```python
from build123d import *
from build123d.topology import SkipClean

# Parameters (mm, degrees)
EXTRUDE_1_DEPTH          = 3
EXTRUDE_3_DEPTH          = 5
EXTRUDE_3_DEPTH_BACK     = 5
SKETCH_5_R               = 6.36543
SKETCH_5_R_2             = 5.5
CUT_EXTRUDE_1_DEPTH      = 14
CUT_EXTRUDE_2_DEPTH      = 15.974979
CUT_EXTRUDE_2_DEPTH_BACK = 15.974979
SKETCH_6_R               = 0.975
SKETCH_7_R               = 3
SKETCH_7_R_2             = 0.9
EXTRUDE_4_DEPTH          = 7.5
CUT_EXTRUDE_3_DEPTH      = 1.45
CUT_EXTRUDE_3_DEPTH_BACK = 1.45
SKETCH_10_R              = 1.825
SKETCH_10_R_2            = 1.025
EXTRUDE_5_DEPTH          = 0.2
SKETCH_11_R              = 3.025
CUT_EXTRUDE_4_DEPTH      = 1.4
SKETCH_12_R              = 4.2
EXTRUDE_6_DEPTH          = 0.4
FILLET_3_R               = 0.3
CHAMFER_1_SIZE           = 0.2
SKETCH_14_R              = 1
CUT_EXTRUDE_5_DEPTH      = 5
SKETCH_15_R              = 0.55
CUT_EXTRUDE_6_DEPTH      = 7


with BuildPart() as part:
    # Sketch 1 → Extrude 1 (new body)
    with BuildSketch(Plane.XY):
        with BuildLine():
            Line((-5, 2.291288), (-5, -2.291288))
            ThreePointArc((-5, -2.291288), (0, -5.5), (5, -2.291288))
            Line((5, -2.291288), (5, 2.291288))
            ThreePointArc((5, 2.291288), (0, 5.5), (-5, 2.291288))
        make_face()
    extrude(amount=EXTRUDE_1_DEPTH)

    # Sketch 4 → Extrude 3 (add, two sides: drawn at the far end of the back side and taken through both)
    with BuildSketch(Plane(origin=(0, 0, 0), x_dir=(0, 0, -1), z_dir=(1, 0, 0)).offset(-EXTRUDE_3_DEPTH_BACK)):
        with BuildLine():
            Line((-3, 3.282066), (-3, -3.282066))
            ThreePointArc((-3, -3.282066), (-6.623628, -3.209089), (-10.241379, -2.990274))
            ThreePointArc((-10.241379, -2.990274), (-13, 0), (-10.241379, 2.990274))
            ThreePointArc((-10.241379, 2.990274), (-6.623628, 3.209089), (-3, 3.282066))
        make_face()
    extrude(amount=EXTRUDE_3_DEPTH + EXTRUDE_3_DEPTH_BACK)

    # Sketch 5 → Cut-Extrude 1 (cut)
    with BuildSketch(Plane(origin=(0, 0, 0), x_dir=(-1, 0, 0), z_dir=(0, 0, -1))):
        Circle(SKETCH_5_R)
        Circle(SKETCH_5_R_2, mode=Mode.SUBTRACT)
    extrude(amount=-CUT_EXTRUDE_1_DEPTH, mode=Mode.SUBTRACT)

    # Sketch 6 → Cut-Extrude 2 (cut, two sides: drawn at the far end of the back side and taken through both)
    with SkipClean():  # the faces are left unmerged after this step: merging them gives an invalid solid
        with BuildSketch(Plane(origin=(0, 0, 0), x_dir=(0, 0, -1), z_dir=(1, 0, 0)).offset(-CUT_EXTRUDE_2_DEPTH_BACK)):
            with Locations((-10, 0)):
                Circle(SKETCH_6_R)
            with Locations((-4, 0)):
                Circle(SKETCH_6_R)
        extrude(amount=CUT_EXTRUDE_2_DEPTH + CUT_EXTRUDE_2_DEPTH_BACK, mode=Mode.SUBTRACT)

    # Sketch 7 → Extrude 4 (add)
    with SkipClean():  # the faces are left unmerged after this step: merging them gives an invalid solid
        with BuildSketch(Plane(origin=(0, 0, 0), x_dir=(-1, 0, 0), z_dir=(0, 0, -1))):
            with Locations(Location((0, 0, 0), (0, 0, 180))):
                Circle(SKETCH_7_R)
            Circle(SKETCH_7_R_2, mode=Mode.SUBTRACT)
        extrude(amount=EXTRUDE_4_DEPTH)

    # Sketch 8 → Cut-Extrude 3 (cut, two sides: drawn at the far end of the back side and taken through both)
    with SkipClean():  # the faces are left unmerged after this step: merging them gives an invalid solid
        with BuildSketch(Plane(origin=(0, 0, 0), x_dir=(0, 0, -1), z_dir=(1, 0, 0)).offset(-CUT_EXTRUDE_3_DEPTH_BACK)):
            with BuildLine():
                ThreePointArc((-4.037779, 3.276083), (-7.142045, 3.186702), (-10.241379, 2.990274))
                ThreePointArc((-10.241379, 2.990274), (-11.143646, 2.773459), (-11.936492, 2.291288))
                ThreePointArc((-11.936492, 2.291288), (-13, 0), (-11.936492, -2.291288))
                ThreePointArc((-11.936492, -2.291288), (-11.143646, -2.773459), (-10.241379, -2.990274))
                ThreePointArc((-10.241379, -2.990274), (-7.142045, -3.186702), (-4.037779, -3.276083))
                add(Edge.make_bspline(
                    [(-6.066615, 0), (-5.84656, -1.308935), (-5.00956, -2.417573), (-4.037779, -3.276083)],
                    knots=[0, 0, 0, 0, 1, 1, 1, 1], degree=3))
                add(Edge.make_bspline(
                    [(-6.066615, 0), (-5.84656, 1.308935), (-5.00956, 2.417573), (-4.037779, 3.276083)],
                    knots=[0, 0, 0, 0, 1, 1, 1, 1], degree=3))
            make_face()
        extrude(amount=CUT_EXTRUDE_3_DEPTH + CUT_EXTRUDE_3_DEPTH_BACK, mode=Mode.SUBTRACT)

    # Sketch 10 → Extrude 5 (add)
    with SkipClean():  # the faces are left unmerged after this step: merging them gives an invalid solid
        with BuildSketch(Plane.ZY.offset(-1.45)):
            with Locations((10, 0)):
                Circle(SKETCH_10_R)
            with Locations((10, 0)):
                Circle(SKETCH_10_R_2, mode=Mode.SUBTRACT)
        extrude_5 = extrude(amount=EXTRUDE_5_DEPTH)

    # Sketch 11 → Cut-Extrude 4 (cut)
    with SkipClean():  # the faces are left unmerged after this step: merging them gives an invalid solid
        with BuildSketch(Plane(origin=(5, 0, 0), x_dir=(0, 0, -1), z_dir=(1, 0, 0))):
            with Locations((-4, 0)):
                Circle(SKETCH_11_R)
        cut_extrude_4 = extrude(amount=-CUT_EXTRUDE_4_DEPTH, mode=Mode.SUBTRACT)

    # Mirror 1: Extrude 5, Cut-Extrude 4 across plane
    with SkipClean():  # the faces are left unmerged after this step: merging them gives an invalid solid
        add(extrude_5.mirror(Plane(origin=(0, 0, 0), x_dir=(0, 0, 1), z_dir=(1, 0, 0))))
        add(cut_extrude_4.mirror(Plane(origin=(0, 0, 0), x_dir=(0, 0, 1), z_dir=(1, 0, 0))), mode=Mode.SUBTRACT)

    # Sketch 12 → Extrude 6 (add)
    with BuildSketch(Plane(origin=(0, 0, 0), x_dir=(-1, 0, 0), z_dir=(0, 0, -1))):
        with Locations(Location((0, 0, 0), (0, 0, 180))):
            Circle(SKETCH_12_R)
    extrude(amount=EXTRUDE_6_DEPTH)

    # Fillet 3
    fillet_3_edges = [part.edges().sort_by_distance(p)[0] for p in [
        (0, 5.5, 3),
        (0, -5.5, 3),
        (0, -5.5, 0),
        (0, 5.5, 0),
    ]]
    fillet(fillet_3_edges, radius=FILLET_3_R)

    # Chamfer 1
    chamfer_1_edges = [part.edges().sort_by_distance(p)[0] for p in [
        (-5, 1.260208, 1.25),
        (-5, 0, 7.025),
        (5, 0, 7.025),
        (5, -1.260208, 1.25),
    ]]
    chamfer(chamfer_1_edges, length=CHAMFER_1_SIZE)

    # Sketch 14 → Cut-Extrude 5 (cut)
    with SkipClean():  # the faces are left unmerged after this step: merging them gives an invalid solid
        with BuildSketch(Plane(origin=(0, -6, 0), x_dir=(1, 0, 0), z_dir=(0, 1, 0))):
            with Locations(Location((0, -1.5, 0), (0, 0, 90))):
                Circle(SKETCH_14_R)
        extrude(amount=CUT_EXTRUDE_5_DEPTH, mode=Mode.SUBTRACT)

    # Sketch 15 → Cut-Extrude 6 (cut)
    with SkipClean():  # the faces are left unmerged after this step: merging them gives an invalid solid
        with BuildSketch(Plane.XZ.offset(1)):
            with Locations(Location((0, 1.5, 0), (0, 0, 270))):
                Circle(SKETCH_15_R)
        extrude(amount=-CUT_EXTRUDE_6_DEPTH, mode=Mode.SUBTRACT)


solid = part.part
```
Geometry check sheet. Reference: the model listing, model coordinates, mm. A direction names the side the tool comes from. Give positions to 0.01 mm unless a question says otherwise; leave off trailing zeros. Loops run counter-clockwise (first coordinate to the right, second up) from the corner with the lowest first, then second, coordinate; pieces in that order, holes last. Notation, with made-up numbers: (32.5, 51) - (85.5, 51) arc R34 ccw to (85.5, 90) - close; hole circle Ø4 at (9, 36). An arc over 180 degrees is marked (long way). Use CSV: the item, a comma, the result in double quotes. Start each with the question number.
Q1. Release check for a two-part mould opening along Y. For faces 1 (the face through (0.976, -3.283, 1.717)), 2 (the face through (-0.86, 0.27, -3.9)), 3 (the face through (0.2, -1, 0.8)), 4 (the face through (3.2, 0.043, 10.974)) record: +Y half, -Y half, draft (parallel to the pull), parting line (faces both ways), or undercut.
Q2. Access from +Z, -Z, +X, -X, +Y, -Y to the whole of each face (thin tool, end or side, straight path). Record for faces 5 (the face through (-1.25, -1, 11)), 6 (the face through (0, -4, 3)), 7 (the face through (3.6, 1, 5)), 8 (the face through (0.165, 2.205, 0.975)), 9 (the face through (4.006, -1.262, -0.197)).
Q3. Go/stop test with flat-tipped pins: pin 1 Ø4 at (x, z) = (1, -3.5) entering from +Y; pin 2 Ø5.5 at (y, z) = (0, 4) entering from -X; pin 3 Ø1.5 at (y, z) = (-1.5, 5) entering from +X; pin 4 Ø1.6 at (y, z) = (0, 10) entering from -X. Record where each tip stops, or that it passes through.
Q4. Section check B-B, the plane z = -4. Record the cut outline in (x, y), and give its area (3 significant figures).
Q5. Section check A-A, the plane x = 0. Count the separate pieces of the cut face and the enclosed holes in it, and give its area (3 significant figures).
Q6. Scan lines: probe 1 along Y at (x, z) = (0.25, 4) (3 decimals); probe 2 along X at (y, z) = (1, 1.5); probe 3 along Z at (x, y) = (0, 2). Record each from-to range of solid material in increasing order. Write a range as from..to.
Findings below:
1,face 1,"draft"
1,face 2,"undercut"
1,face 3,"-Y half"
1,face 4,"undercut"
2,face 5,"+Z, +Y, -Y"
2,face 6,"+Z, +X, -X, -Y"
2,face 7,"+X"
2,face 8,"+Y, -Y"
2,face 9,"-Z"
3,pin 1,"stops at y = 3"
3,pin 2,"stops at x = -3.6"
3,pin 3,"stops at x = 3.6"
3,pin 4,"passes through"
4,outline,"circle Ø6 at (0, 0); hole circle Ø1.8 at (0, 0)"
4,area,"25.7 mm^2"
5,separate pieces,"2"
5,enclosed holes,"1"
5,area,"62.1 mm^2"
6,probe 1,"y = -3.277..-0.975, 0.975..3.277"
6,probe 2,"x = -3.6..-0.55, 0.55..3.6"
6,probe 3,"z = -7.5..0.95, 2.05..5.2"
